CAD build for the part. Positions are in the model's coordinates, mm. Face numbers are marked on the shaded views. A direction names the side the tool comes from. Give positions to 0.01 mm unless a question says otherwise; leave off trailing zeros. Loops run counter-clockwise (first coordinate to the right, second up) from the corner with the lowest first, then second, coordinate; pieces in that order, holes last. Notation, with made-up numbers: (6.25, 1) - (57.25, 1) arc R27 ccw to (57.25, 25) - close; hole circle Ø3 at (56.25, -6.75). An arc over 180 degrees is marked (long way). Return JSON: item names as keys, results as strings.
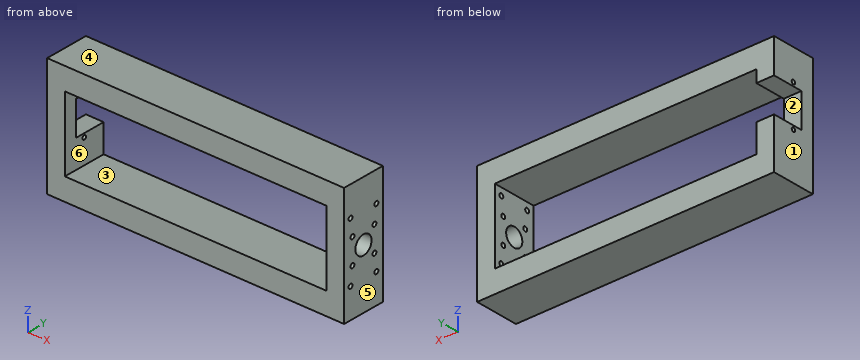
from build123d import *

# Parameters (mm, degrees)
SKETCH1_W           = 201.19
SKETCH1_H           = 80
SKETCH1_W_2         = 177.19
SKETCH1_H_2         = 50
BOSS_EXTRUDE1_DEPTH = 30
SKETCH2_R           = 1.35
SKETCH2_W           = 22.92
SKETCH2_H           = 21.2
CUT_EXTRUDE1_DEPTH  = 30
SKETCH4_R           = 6.25
SKETCH4_R_2         = 1.52
CUT_EXTRUDE2_DEPTH  = 30


with BuildPart() as part:
    # Sketch1 → Boss-Extrude1 (new body)
    with BuildSketch(Plane(origin=(0, 0, 0), x_dir=(1, 0, 0), z_dir=(0, 1, 0))):
        with Locations((30.629887821, -19.526338141)):
            Rectangle(SKETCH1_W, SKETCH1_H)
        with Locations((30.629887821, -19.526338141)):
            Rectangle(SKETCH1_W_2, SKETCH1_H_2, mode=Mode.SUBTRACT)
    extrude(amount=BOSS_EXTRUDE1_DEPTH)

    # Sketch2 → Cut-Extrude1 (cut)
    with BuildSketch(Plane.ZY.offset(69.965112179)):
        with Locations((10.926338141, 15)):
            Circle(SKETCH2_R)
        with Locations((38.926338141, 15)):
            Circle(SKETCH2_R)
        with Locations((24.926338141, 19.4)):
            Rectangle(SKETCH2_W, SKETCH2_H)
    extrude(amount=-CUT_EXTRUDE1_DEPTH, mode=Mode.SUBTRACT)

    # Sketch4 → Cut-Extrude2 (cut)
    with BuildSketch(Plane(origin=(131.224887821, 0, 0), x_dir=(0, 0, -1), z_dir=(1, 0, 0))):
        with Locations((-19.526338141, 15)):
            Circle(SKETCH4_R)
        with Locations((-28.026338141, 23.5)):
            Circle(SKETCH4_R_2)
        with Locations((-11.026338141, 23.5)):
            Circle(SKETCH4_R_2)
        with Locations((-11.026338141, 6.5)):
            Circle(SKETCH4_R_2)
        with Locations((-28.026338141, 6.5)):
            Circle(SKETCH4_R_2)
        with Locations((0.473661859, 25)):
            Circle(SKETCH4_R_2)
        with Locations((0.473661859, 5)):
            Circle(SKETCH4_R_2)
        with Locations((-39.526338141, 5)):
            Circle(SKETCH4_R_2)
        with Locations((-39.526338141, 25)):
            Circle(SKETCH4_R_2)
    extrude(amount=-CUT_EXTRUDE2_DEPTH, mode=Mode.SUBTRACT)


solid = part.part
1. Cut at B-B, the plane x = 66. Write the cut outline in (y, z).
Values follow:
{"outline": "(0, -20.47) - (30, -20.47) - (30, -5.47) - (0, -5.47) - close; (0, 44.53) - (30, 44.53) - (30, 59.53) - (0, 59.53) - close"}
2. Cut at A-A, the plane y = 11.25. Write the cut outline in (x, z).
Values follow:
{"outline": "(-69.97, -20.47) - (131.22, -20.47) - (131.22, 14.53) - (119.22, 14.53) - (119.22, -5.47) - (-57.97, -5.47) - (-57.97, 13.47) - (-69.97, 13.47) - close; (-69.97, 36.39) - (-57.97, 36.39) - (-57.97, 44.53) - (119.22, 44.53) - (119.22, 24.53) - (131.22, 24.53) - (131.22, 59.53) - (-69.97, 59.53) - close"}
3. Cut at C-C, the plane z = 21. Write the cut outline in (x, y), plus the area to 3 significant figures.
Values follow:
{"outline": "(-69.97, 0) - (-57.97, 0) - (-57.97, 8.8) - (-69.97, 8.8) - close; (119.22, 0) - (131.22, 0) - (131.22, 8.93) - (119.22, 8.93) - close; (119.22, 21.07) - (131.22, 21.07) - (131.22, 30) - (119.22, 30) - close", "area": "320 mm²"}
4. Drill centre lines: probe 1 along Z at (x, y) = (65.5, 15.75); probe 2 along X at (y, z) = (13, -3.5); probe 3 along X at (y, z) = (15.5, 29). Where is each one in solid material? Low to high.
Values follow:
{"probe 1": "z = -20.47 to -5.47, 44.53 to 59.53", "probe 2": "x = -69.97 to -57.97, 119.22 to 131.22", "probe 3": "x = 119.22 to 131.22"}
5. Drop flat-ended pins along their axis: P1, Ø9.5, axis at x = -65.5, z = 26.5, coming from the +Y side; P2, Ø2, axis at y = 16, z = 34.5, coming from the -X side; P3, Ø2.5, axis at y = 25, z = 39.53, coming from the +X side. Give the stop position or say it passes through.
Values follow:
{"P1": "stops at y = 8.8", "P2": "stops at x = 119.22", "P3": "stops at x = -57.97"}
6. Pull direction Z, two halves, no side cores. Call the marked faces 4, 5 and 6: +Z half, -Z half, draft (parallel to the pull), parting line (faces both ways), or undercut.
Values follow:
{"face 4": "+Z half", "face 5": "draft", "face 6": "undercut"}
7. Which spindle directions (+Z, -Z, +X, -X, +Y, -Y) get a long thin tool onto all of the face, cutting with end or side? Do the marked faces 1, 2 and 3. Say none if no direction does.
Values follow:
{"face 1": "+Z, -Z, -X, +Y, -Y", "face 2": "-X, +Y", "face 3": "+Y, -Y"}
